from build123d import *

# Parameters (mm, degrees)
BOSS_EXTRUDE1_DEPTH         = 12.7
F_1_4_0_25_DIAMETER_HOLE1_D = 6.35
CHAMFER1_SIZE               = 7.9375
SKETCH6_R                   = 7.9375
CUT_EXTRUDE1_DEPTH          = 10.525
SKETCH7_R                   = 12.7
CUT_EXTRUDE2_DEPTH          = 26.4


with BuildPart() as part:
    # Sketch1 → Boss-Extrude1 (new body, symmetric)
    with BuildSketch(Plane.XY):
        Polygon((6.35, 12.7), (44.45, 12.7), (44.45, 7.9375), (15.875, 7.9375), (15.875, -7.9375), (44.45, -7.9375), (44.45, -12.7), (6.35, -12.7), align=None)
    extrude(amount=BOSS_EXTRUDE1_DEPTH, both=True)

    # 1/4 (0.25) Diameter Hole1 (through all)
    with Locations(Plane(origin=(0, 12.7, 0), x_dir=(1, 0, 0), z_dir=(0, 1, 0))):
        with Locations((38.1, 0)):
            Hole(F_1_4_0_25_DIAMETER_HOLE1_D / 2)

    # Chamfer1
    chamfer1_edges = [part.edges().sort_by_distance(p)[0] for p in [
        (44.45, 10.31875, 12.7),
        (44.45, -10.31875, 12.7),
        (44.45, -10.31875, -12.7),
        (44.45, 10.31875, -12.7),
    ]]
    chamfer(chamfer1_edges, length=CHAMFER1_SIZE)

    # Sketch6 → Cut-Extrude1 (cut, through all)
    with BuildSketch(Plane(origin=(15.875, 0, 0), x_dir=(0, 0, -1), z_dir=(1, 0, 0))):
        Circle(SKETCH6_R)
    extrude(amount=-CUT_EXTRUDE1_DEPTH, mode=Mode.SUBTRACT)

    # Sketch7 → Cut-Extrude2 (cut, through all)
    with BuildSketch(Plane(origin=(0, 12.7, 0), x_dir=(1, 0, 0), z_dir=(0, 1, 0))):
        Circle(SKETCH7_R)
    extrude(amount=-CUT_EXTRUDE2_DEPTH, mode=Mode.SUBTRACT)


solid = part.part
The listing builds one solid part. Answer for the finished solid, in the listing's coordinates (mm). A direction names the side the tool comes from. Give positions to 0.01 mm unless a question says otherwise; leave off trailing zeros. Order: outer loops, then holes, each group sorted by start corner. A loop starts at its lowest first (then second) coordinate and runs counter-clockwise, first axis right, second up. Notation, with made-up numbers: (24, -38) - (70, -38) arc R17 cw to (70, -12) - close; hole circle Ø3 at (8, 85.25). An arc over 180 degrees is marked (long way). One line per item, written item: value. Start each with the question number.
1) The mould has two halves that part along X. Classify faces 1 (the face through (40.537, -10.285, -8.676)), 2 (the face through (11.26, 5.82, 5.87)), 3 (the face through (41.27, -10.35, -0.14)): released by +X, released by -X, zero draft, split by the parting line, or undercut.
2) A cutting plane is placed at B-B on x = 19. Give the vertices of the cut face in (y, z).
3) A tool of negligible diameter and unlimited length cuts with its end or side. For faces 4 (the face through (44.45, 10, 0)), 5 (the face through (15.875, 0, -9)), from which of +Z, -Z, +X, -X, +Y, -Y can it reach the whole face along a straight path? Write none if from no direction.
4) Find the intervals of material crossed by L1, parallel to Z at x = 11.5, y = 0; L2, parallel to Z at x = 38.1, y = 9.5 (1 decimal), in increasing order.
5) Given pin 1 Ø6.5 at (y, z) = (3.5, 4) entering from +X (3 decimals); pin 2 Ø5.5 at (x, z) = (38.1, 0) entering from +Y; pin 3 Ø1.5 at (y, z) = (9, 8.5) entering from -X, each flat-ended and moving along its own axis, determine where each tip first touches the part or whether it passes through.
6) A cutting plane is placed at D-D on x = 14. Give the vertices of the cut face in (y, z) (1 decimal), then the cut area to 3 significant figures.
Answer sheet:
1. face 1: released by +X
1. face 2: released by -X
1. face 3: undercut
2. outline: (-12.7, -12.7) - (-7.94, -12.7) - (-7.94, 12.7) - (-12.7, 12.7) - close; (7.94, -12.7) - (12.7, -12.7) - (12.7, 12.7) - (7.94, 12.7) - close
3. face 4: +Z, -Z, +X, +Y, -Y
3. face 5: +Z, -Z, +X
4. L1: z = -12.7 to -7.94, 7.94 to 12.7
4. L2: z = -11.1 to -3.2, 3.2 to 11.1
5. pin 1: stops at x = 15.875
5. pin 2: passes through
5. pin 3: stops at x = 8.7
6. outline: (-12.7, -12.7) - (12.7, -12.7) - (12.7, 12.7) - (-12.7, 12.7) - close; hole circle Ø15.9 at (0, 0)
6. area: 447 mm2
